Design review of the part built by this model. Coordinates are the model's own, in mm. Give positions to 0.01 mm unless a question says otherwise; leave off trailing zeros. Loops run counter-clockwise (first coordinate to the right, second up) from the corner with the lowest first, then second, coordinate; pieces in that order, holes last. Notation, with made-up numbers: (28, 75.25) - (66, 75.25) arc R38 cw to (66, 113.25) - close; hole circle Ø3 at (51.25, -2). An arc over 180 degrees is marked (long way). Write each question's results on one line, items separated by ' | '.
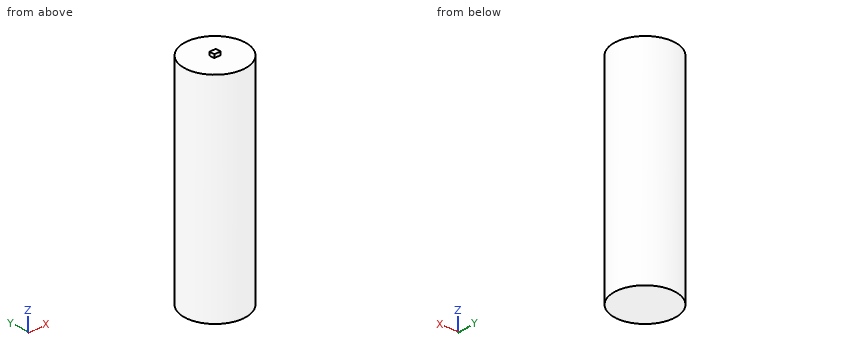
from build123d import *

# Parameters (mm, degrees)
SKETCH_1_R      = 9.3
EXTRUDE_1_DEPTH = 32.6
SKETCH_2_W      = 2
SKETCH_2_H      = 1.651721756
EXTRUDE_2_DEPTH = 1


with BuildPart() as part:
    # Эскиз1 → Бобышка-Вытянуть1 (new, symmetric)
    with BuildSketch(Plane.XY):
        Circle(SKETCH_1_R)
    extrude(amount=EXTRUDE_1_DEPTH, both=True)

    # Эскиз2 → Бобышка-Вытянуть2 (add)
    with BuildSketch(Plane.XY.offset(32.6)):
        Rectangle(SKETCH_2_W, SKETCH_2_H)
    extrude(amount=EXTRUDE_2_DEPTH)


solid = part.part
(1) Take a section at C-C on x = 2.5. Give the boundary of the cut face in (y, z), plus the area to 3 significant figures.
Answers below:
outline: (-8.96, -32.6) - (8.96, -32.6) - (8.96, 32.6) - (-8.96, 32.6) - close | area: 1,170 mm2
(2) Take a section at B-B on y = -4. Give the boundary of the cut face in (x, z), plus the area to 3 significant figures.
Answers below:
outline: (-8.4, -32.6) - (8.4, -32.6) - (8.4, 32.6) - (-8.4, 32.6) - close | area: 1,090 mm2
(3) Take a section at A-A on z = 25. Give the boundary of the cut face in (x, y), plus the area to 3 significant figures.
Answers below:
outline: circle Ø18.6 at (0, 0) | area: 272 mm2
(4) Insertion check: P1, Ø8, axis at x = 4.5, z = -7, coming from the +Y side; P2, Ø1, axis at x = 6.5, z = 25, coming from the -Y side; P3, Ø1, axis at x = -1.5, z = 5.5, coming from the +Y side; P4, Ø1.1, axis at y = 0, z = 33, coming from the -X side. Each pin has a flat end and moves straight along its axis. Give the tip position at first contact, or say it passes through.
Answers below:
P1: y = 9.29 | P2: y = -7.11 | P3: y = 9.25 | P4: x = -9.3
(5) Wall thickness on line 1 along Z through (x, y) = (3, -3); line 2 along X through (y, z) = (0.5, 4); line 3 along Y through (x, z) = (-3, 15.5): over which ranges is each line inside the solid? List them lowest first. Write a range as from..to.
Answers below:
line 1: -32.6..32.6 | line 2: -9.29..9.29 | line 3: -8.8..8.8
